Input: part model. Units: mm. Frame: model coordinates. A direction names the side the tool comes from. Give positions to 0.01 mm unless a question says otherwise; leave off trailing zeros. Write each loop counter-clockwise with the first axis right and the second up, starting at its lowest first coordinate (ties: lowest second). Pieces come first, ordered by that corner, then holes. Notation, with made-up numbers: (23, 44) -> (38, 44) arc R22 ccw to (38, 62) -> close; hole circle Ø8 at (13.5, 50.5). An arc over 180 degrees is marked (long way). Answer as a JSON object with one key per item and string values. Group by question number.
from build123d import *

# Parameters (mm, degrees)
SKETCH1_W           = 90
SKETCH1_H           = 60
BOSS_EXTRUDE1_DEPTH = 3
BOSS_EXTRUDE2_DEPTH = 2
SKETCH4_W           = 30
SKETCH4_H           = 60
BOSS_EXTRUDE4_DEPTH = 3
SKETCH5_R           = 0.9
CUT_EXTRUDE1_DEPTH  = 22
SKETCH6_W           = 10
SKETCH6_H           = 25
CUT_EXTRUDE2_DEPTH  = 9
FILLET1_R           = 15
CUT_EXTRUDE3_DEPTH  = 4


with BuildPart() as part:
    # Sketch1 → Boss-Extrude1 (new body)
    with BuildSketch(Plane(origin=(0, 0, 0), x_dir=(1, 0, 0), z_dir=(0, 1, 0))):
        Rectangle(SKETCH1_W, SKETCH1_H)
    extrude(amount=-BOSS_EXTRUDE1_DEPTH)

    # Sketch2 → Boss-Extrude2 (add)
    with BuildSketch(Plane(origin=(0, 0, 0), x_dir=(1, 0, 0), z_dir=(0, 1, 0))):
        Polygon((45, 30), (-45, 30), (-45, 27.5), (-45, -27.5), (-45, -30), (45, -30), align=None)
        Polygon((43, 0), (23.02008048, 27.5), (-15, 27.5), (-15, -27.5), (23.02008048, -27.5), align=None, mode=Mode.SUBTRACT)
    extrude(amount=BOSS_EXTRUDE2_DEPTH)

    # Sketch4 → Boss-Extrude4 (add)
    with BuildSketch(Plane(origin=(0, 2, 0), x_dir=(1, 0, 0), z_dir=(0, 1, 0))):
        with Locations((-30, 0)):
            Rectangle(SKETCH4_W, SKETCH4_H)
    extrude(amount=BOSS_EXTRUDE4_DEPTH)

    # Sketch5 → Cut-Extrude1 (cut)
    with BuildSketch(Plane(origin=(-15, 0, 0), x_dir=(0, 0, -1), z_dir=(1, 0, 0))):
        with Locations((0, 1.5)):
            Circle(SKETCH5_R)
        with Locations((6, 1.5)):
            Circle(SKETCH5_R)
        with Locations((12, 1.5)):
            Circle(SKETCH5_R)
    extrude(amount=-CUT_EXTRUDE1_DEPTH, mode=Mode.SUBTRACT)

    # Sketch6 → Cut-Extrude2 (cut, through all)
    with BuildSketch(Plane(origin=(0, 5, 0), x_dir=(1, 0, 0), z_dir=(0, 1, 0))):
        with Locations((-30, 7.5)):
            Rectangle(SKETCH6_W, SKETCH6_H)
    extrude(amount=-CUT_EXTRUDE2_DEPTH, mode=Mode.SUBTRACT)

    # Fillet1
    fillet1_edges = [part.edges().sort_by_distance(p)[0] for p in [
        (-45, 1, -30),
        (-45, 1, 30),
        (45, -0.5, 30),
        (45, -0.5, -30),
    ]]
    fillet(fillet1_edges, radius=FILLET1_R)

    # Sketch7 → Cut-Extrude3 (cut, through all)
    with BuildSketch(Plane(origin=(0, 0, 0), x_dir=(1, 0, 0), z_dir=(0, 1, 0))):
        Polygon((35.541019662, 0), (22.729490169, 17.633557569), (2, 10.89813792), (2, -10.89813792), (22.729490169, -17.633557569), align=None)
    extrude(amount=-CUT_EXTRUDE3_DEPTH, mode=Mode.SUBTRACT)


solid = part.part
1. Section B-B (x = -33). Return the cut outline in (y, z), plus the area to 3 significant figures.
2. Section C-C (y = 3.5). Return the cut outline in (x, z).
3. Section D-D (z = -9). Return the cut outline in (x, y).
4. Contact query for flat-ended pins moving along their axis: pin 1 Ø1.5 at (x, z) = (3.5, -17.5) entering from +Y; pin 2 Ø4 at (x, y) = (35, 2) entering from +Z; pin 3 Ø5 at (x, z) = (-33.5, -16.5) entering from -Y. Output: stop coordinate, or through.
5. Line query: line 1 (Y direction, x = -18.5, z = -12); line 2 (X direction, y = 0.5, z = 3); line 3 (X direction, y = 1.75, z = -3.5). Output: solid intervals per line, ascending.
6. Mould query, pull axis Y, two halves, no side actions, for faces 4 (the face through (-35.99, 1.77, -12.86)), 5 (the face through (1, 0, 0)), 6 (the face through (29, -1, 9)). Classes: pulls with the +Y half, pulls with the -Y half, needs draft (parallel to the pull), parting line crosses it, or undercut.
7. Section A-A (y = -1.75). Return the cut outline in (x, z), plus the area to 3 significant figures.
8. Reachability of faces 1 (the face through (-35.99, 2.39, 0.12)), 2 (the face through (12.51, -1.479, -14.313)), 3 (the face through (4, 1, -27.5)) from +Z, -Z, +X, -X, +Y, -Y: full face, straight path, thin tool, end or side. Return the list, or none.
Working result:
{
 "1": {"outline": "(-3, -29.7) -> (5, -29.7) -> (5, -20) -> (-3, -20) -> close; (-3, 5) -> (5, 5) -> (5, 29.7) -> (-3, 29.7) -> close", "area": "275 mm^2"},
 "2": {"outline": "(-45, -15) arc R15 ccw to (-30, -30) -> (-15, -30) -> (-15, 30) -> (-30, 30) arc R15 ccw to (-45, 15) -> close; hole (-35, -20) -> (-25, -20) -> (-25, 5) -> (-35, 5) -> close"},
 "3": {"outline": "(-45, -3) -> (-35, -3) -> (-35, 5) -> (-45, 5) -> close; (-25, -3) -> (2, -3) -> (2, 0) -> (-15, 0) -> (-15, 5) -> (-25, 5) -> close; (29, -3) -> (45, -3) -> (45, 2) -> (36.46, 2) -> (36.46, 0) -> (29, 0) -> close"},
 "4": {"pin 1": "stops at y = 0", "pin 2": "stops at z = 29.7", "pin 3": "stops at y = -3"},
 "5": {"line 1": "y = -3 to 0.6, 2.4 to 5", "line 2": "x = -45 to -35, -25 to -15, 40.82 to 45", "line 3": "x = -45 to -35, -25 to -15, 40.46 to 45"},
 "6": {"face 4": "undercut", "face 5": "pulls with the +Y half", "face 6": "needs draft"},
 "7": {"outline": "(-45, -15) arc R15 ccw to (-30, -30) -> (30, -30) arc R15 ccw to (45, -15) -> (45, 15) arc R15 ccw to (30, 30) -> (-30, 30) arc R15 ccw to (-45, 15) -> close; hole (-35, -20) -> (-25, -20) -> (-25, 5) -> (-35, 5) -> close; hole (2, -10.9) -> (22.73, -17.63) -> (35.54, 0) -> (22.73, 17.63) -> (2, 10.9) -> close", "area": "4,140 mm^2"},
 "8": {"face 1": "none", "face 2": "+Y, -Y", "face 3": "+Y"}
}
